Verification items for this drawing (mm, ordinates from the low corner). A direction names the side the tool comes from. Coordinates: 2 decimals unless noted, no trailing zeros. Write each loop counter-clockwise with the first axis right and the second up, starting at its lowest first coordinate (ties: lowest second). Pieces come first, ordered by that corner, then holes. Notation, with made-up numbers: (-0.5, 17.5) -> (29.5, 17.5) arc R25 cw to (29.5, 56.5) -> close; hole circle Ø4 at (55.25, -34). An arc over 180 degrees is marked (long way). Put each result on its own line as item: value. Start each with the question number.
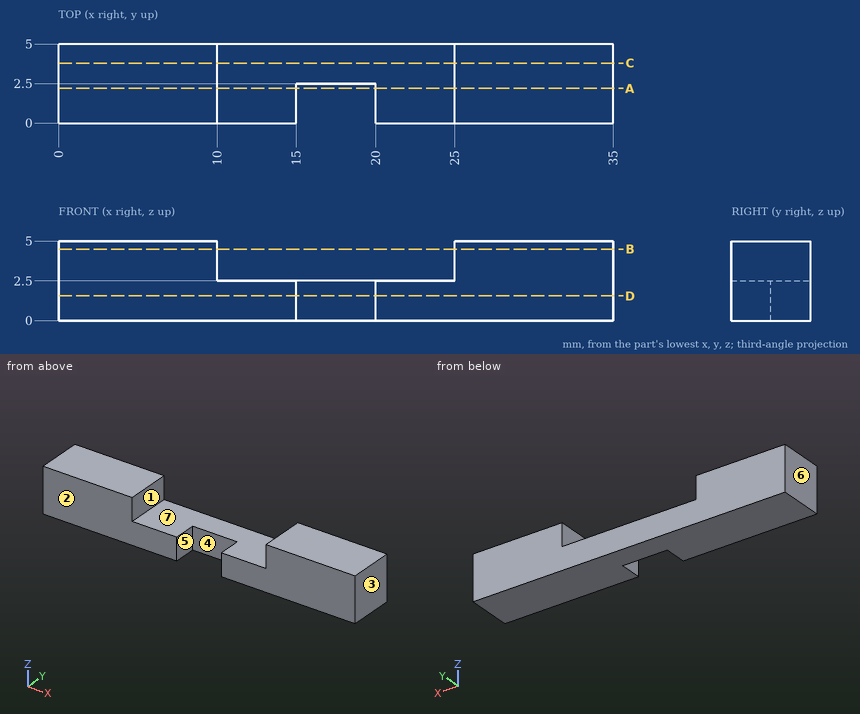
Item 1: Mould release check, pull along X, two halves, no side actions. Record for the marked faces 1, 2, 3 and 4: released by +X, released by -X, zero draft, split by the parting line, or undercut.
Item 2: Section check A-A, the plane y = 2.2. Enter the section's corners in (x, z).
Item 3: Section check B-B, the plane z = 4.5. Enter the section's corners in (x, y).
Item 4: Scan lines: line 1 along X through (y, z) = (0.5, 2.6); line 2 along X through (y, z) = (0.65, 2.05); line 3 along Z through (x, y) = (10.5, 2.6). Record each from-to range of solid material in increasing order. Write a range as [from, to].
Item 5: Access from +Z, -Z, +X, -X, +Y, -Y to the whole of each face (thin tool, end or side, straight path). Record for the marked faces 5, 6 and 7.
Item 6: Section check D-D, the plane z = 1.55. Enter the section's corners in (x, y).
Item 7: Go/stop test with flat-tipped pins: P1, Ø1.5, axis at x = 16, y = 2, coming from the +Z side; P2, Ø0.8, axis at x = 16.5, z = 1.5, coming from the -Y side. Record where each tip stops, or that it passes through.
Item 8: Section check C-C, the plane y = 3.8. Enter the section's corners in (x, z).
From the geometry:
1. face 1: undercut
1. face 2: zero draft
1. face 3: released by +X
1. face 4: undercut
2. outline: (0, 0) -> (15, 0) -> (15, 2.5) -> (10, 2.5) -> (10, 5) -> (0, 5) -> close; (20, 0) -> (35, 0) -> (35, 5) -> (25, 5) -> (25, 2.5) -> (20, 2.5) -> close
3. outline: (0, 0) -> (10, 0) -> (10, 5) -> (0, 5) -> close; (25, 0) -> (35, 0) -> (35, 5) -> (25, 5) -> close
4. line 1: [0, 10], [25, 35]
4. line 2: [0, 15], [20, 35]
4. line 3: [0, 2.5]
5. face 5: +Z, -Z, -Y
5. face 6: +Z, -Z, -X, +Y, -Y
5. face 7: +Z, +Y, -Y
6. outline: (0, 0) -> (15, 0) -> (15, 2.5) -> (20, 2.5) -> (20, 0) -> (35, 0) -> (35, 5) -> (0, 5) -> close
7. P1: z = 2.5
7. P2: y = 2.5
8. outline: (0, 0) -> (35, 0) -> (35, 5) -> (25, 5) -> (25, 2.5) -> (10, 2.5) -> (10, 5) -> (0, 5) -> close
